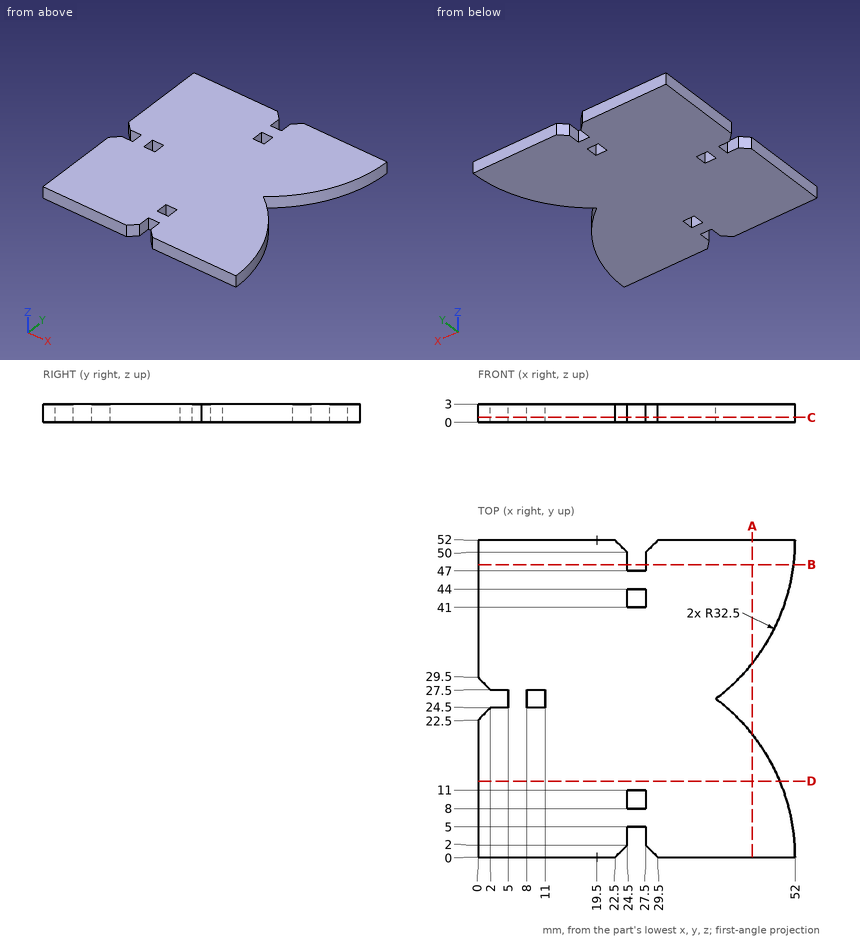
Here's the drawing with two shaded views (mm, measured from the low corner). I have some questions. Give positions to 0.01 mm unless a question says otherwise; leave off trailing zeros. Order: outer loops, then holes, each group sorted by start corner. A loop starts at its lowest first (then second) coordinate and runs counter-clockwise, first axis right, second up. Notation, with made-up numbers: M -39.5,-20 L -22.5,-20 A13 ccw -22.5,0 Z; hole C 54,-20.75 d11. An arc over 180 degrees is marked long. One line per item, written item: value.
1) I want a section at B-B, the plane y = 48. List the corners of the cut face in (x, z) for me.
Answer sheet:
outline: M 0,0 L 24.5,0 L 24.5,3 L 0,3 Z; M 27.5,0 L 51.75,0 L 51.75,3 L 27.5,3 Z
2) I want a section at A-A, the plane x = 45. List the corners of the cut face in (y, z) for me, plus the area to 3 significant figures.
Answer sheet:
outline: M 0,0 L 20.15,0 L 20.15,3 L 0,3 Z; M 31.85,0 L 52,0 L 52,3 L 31.85,3 Z
area: 121 mm^2
3) Please list where these lines run through material, in increasing order: line 1 along Y through (x, z) = (25.5, 1.25); line 2 along Y through (x, z) = (9.5, 0.7); line 3 along Y through (x, z) = (43.5, 2.35).
Answer sheet:
line 1: y = 5 to 8, 11 to 41, 44 to 47
line 2: y = 0 to 24.5, 27.5 to 52
line 3: y = 0 to 21.91, 30.09 to 52
4) I want a section at D-D, the plane y = 12.5. List the corners of the cut face in (x, z) for me, plus the area to 4 significant figures.
Answer sheet:
outline: M 0,0 L 49.5,0 L 49.5,3 L 0,3 Z
area: 148.5 mm^2
5) For P1, Ø1, axis at y = 28.5, z = 2.5, coming from the +X side; P2, Ø1.5, axis at x = 26.5, z = 1.5, coming from the +Y side; P3, Ø1.5, axis at y = 35, z = 1, coming from the +X side, each with a flat end and sliding along its axis, tell me the tip position at first contact or that it passes through.
Answer sheet:
P1: stops at x = 42.46
P2: stops at y = 47
P3: stops at x = 47.65
6) I want a section at C-C, the plane z = 0.8. Count the separate pieces of the cut face and the enclosed holes in it, plus the area to 3 significant figures.
Answer sheet:
separate pieces: 1
enclosed holes: 3
area: 2,420 mm^2
